The figure shows three views and two pictorial views of one solid part (mm, origin at its lowest corner). Answer the questions. A direction names the side the tool comes from. Give positions to 0.01 mm unless a question says otherwise; leave off trailing zeros. Write each loop counter-clockwise with the first axis right and the second up, starting at its lowest first coordinate (ties: lowest second). Pieces come first, ordered by that corner, then holes. Notation, with made-up numbers: (59, 40) -> (118, 40) arc R17 ccw to (118, 59) -> close; hole circle Ø2 at (30.5, 86.25). An arc over 180 degrees is marked (long way). Use a Markdown table: item, result.
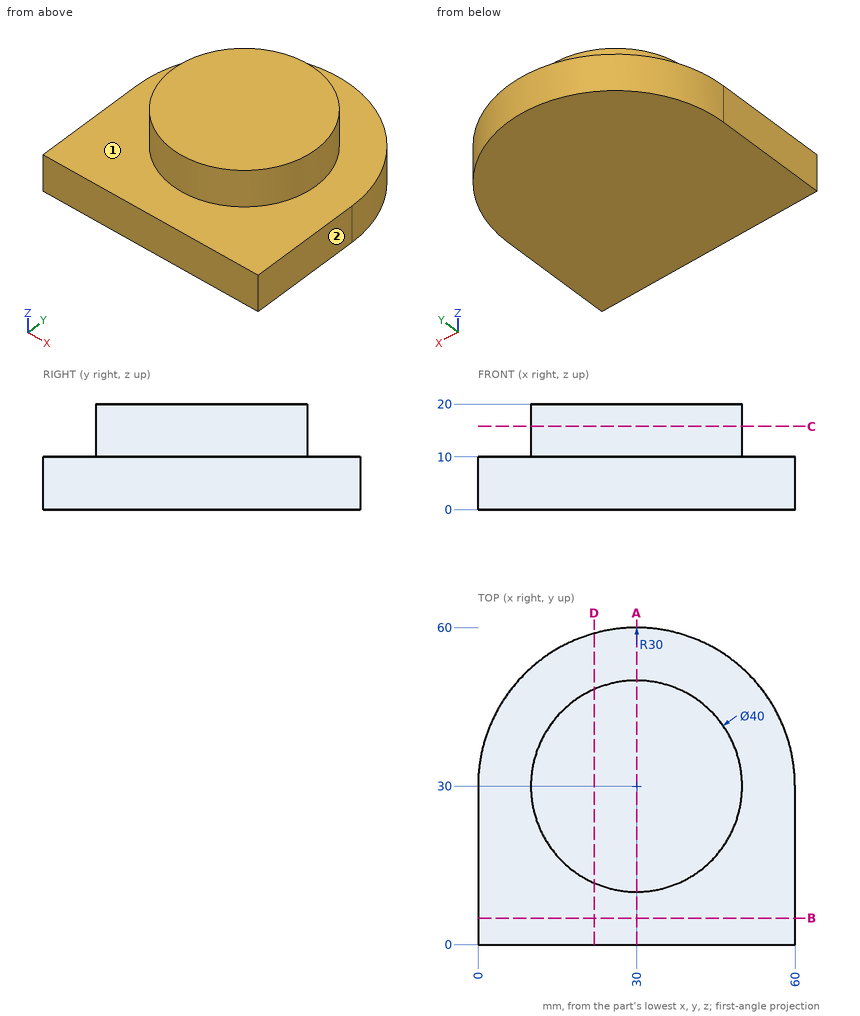
Item 1: A tool of negligible diameter and unlimited length cuts with its end or side. For the marked faces 1 and 2, from which of +Z, -Z, +X, -X, +Y, -Y can it reach the whole face along a straight path? Write none if from no direction.
Return value:
| item | result |
|---|---|
| face 1 | +Z |
| face 2 | +Z, -Z, +X, +Y, -Y |
Item 2: Each of these flat-tipped pins is pushed along its axis until it touches: P1, Ø2, axis at x = 35.5, z = 15.5, coming from the +Y side; P2, Ø1, axis at x = 36.5, z = 16, coming from the +Y side. Where does it stop, or does it pass through?
Return value:
| item | result |
|---|---|
| P1 | y = 49.49 |
| P2 | y = 49.08 |
Item 3: A cutting plane is placed at D-D (x = 22). Give the vertices of the cut face in (y, z), then the cut area to 3 significant figures.
Return value:
| item | result |
|---|---|
| outline | (0, 0) -> (58.91, 0) -> (58.91, 10) -> (48.33, 10) -> (48.33, 20) -> (11.67, 20) -> (11.67, 10) -> (0, 10) -> close |
| area | 956 mm^2 |
Item 4: Straight lines are drawn through the part: line 1 along Z through (x, y) = (9.5, 11.5); line 2 along X through (y, z) = (51, 6); line 3 along Y through (x, z) = (22, 12.25). For each, find the intervals that lie inside material, in ascending order. Write a range as [from, to].
Return value:
| item | result |
|---|---|
| line 1 | [0, 10] |
| line 2 | [8.58, 51.42] |
| line 3 | [11.67, 48.33] |
Item 5: A cutting plane is placed at A-A (x = 30). Give the vertices of the cut face in (y, z), then the cut area to 3 significant figures.
Return value:
| item | result |
|---|---|
| outline | (0, 0) -> (60, 0) -> (60, 10) -> (50, 10) -> (50, 20) -> (10, 20) -> (10, 10) -> (0, 10) -> close |
| area | 1,000 mm^2 |
Item 6: A cutting plane is placed at C-C (z = 15.75). Give the vertices of the cut face in (x, y), then the cut area to 3 significant figures.
Return value:
| item | result |
|---|---|
| outline | circle Ø40 at (30, 30) |
| area | 1,260 mm^2 |
Item 7: A cutting plane is placed at B-B (y = 5). Give the vertices of the cut face in (x, z).
Return value:
| item | result |
|---|---|
| outline | (0, 0) -> (60, 0) -> (60, 10) -> (0, 10) -> close |
